```python
from build123d import *

# Parameters (mm, degrees)
BOSS_EXTRUDE1_DEPTH = 200
SKETCH2_W           = 11
SKETCH2_H           = 5
CUT_EXTRUDE1_DEPTH  = 10
FILLET1_R           = 9
MIRROR1_START       = 184
MIRROR1_DEPTH       = 11


with BuildPart() as part:
    # Sketch1 → Boss-Extrude1 (new body)
    with BuildSketch(Plane(origin=(0, 0, 0), x_dir=(0, 0, -1), z_dir=(1, 0, 0))):
        with BuildLine():
            Line((-9.5, 0), (-9.5, -9.5))
            ThreePointArc((-9.5, -9.5), (0, -19), (9.5, -9.5))
            Line((9.5, -9.5), (9.5, 0))
            ThreePointArc((9.5, 0), (0, 9.5), (-9.5, 0))
        make_face()
    extrude(amount=BOSS_EXTRUDE1_DEPTH)

    # Sketch2 → Cut-Extrude1 (cut, symmetric)
    with BuildSketch(Plane.XY):
        with Locations((10.5, -16.5)):
            Rectangle(SKETCH2_W, SKETCH2_H)
    extrude(amount=CUT_EXTRUDE1_DEPTH, both=True, mode=Mode.SUBTRACT)

    # Fillet1
    # the kernel refuses this fillet: 9 mm, written as the material it takes off along each edge
    with BuildSketch(Plane(origin=(16, -14, -8.366600265), x_dir=(0, 0.9921634898396948, -0.12494642623587741), z_dir=(-1, 0, 0))) as fillet1_piece_1:
        with BuildLine():
            CenterArc((7.946567819, -8.929471409), FILLET1_R, 82.822338024, 90)
            Line((-0.98290359, -7.804953572), (-1.875850731, -7.692501789))
            Line((-1.875850731, -7.692501789), (-0.892947141, 0.112451784))
            Line((-0.892947141, 0.112451784), (-0.323939264, 0.839680507))
            ThreePointArc((-0.323939264, 0.839680507), (4.718801734, 1.455206059), (9.183537439, 0.892947141))
            Line((9.183537439, 0.892947141), (9.071085655, 0))
        make_face()
    extrude(amount=11, mode=Mode.SUBTRACT)
    with BuildSketch(Plane(origin=(16, -14, 8.366600265), x_dir=(0, 0.9921634898396948, 0.1249464262358778), z_dir=(-1, 0, 0))) as fillet1_piece_2:
        with BuildLine():
            CenterArc((7.946567819, 8.929471409), FILLET1_R, 187.177661976, 90)
            Line((-0.98290359, 7.804953572), (-1.875850731, 7.692501789))
            Line((-1.875850731, 7.692501789), (-0.892947141, -0.112451784))
            Line((-0.892947141, -0.112451784), (-0.323939264, -0.839680507))
            ThreePointArc((-0.323939264, -0.839680507), (4.718801734, -1.455206059), (9.183537439, -0.892947141))
            Line((9.183537439, -0.892947141), (9.071085655, 0))
        make_face()
    extrude(amount=11, mode=Mode.SUBTRACT)

    # Mirror1: read off the stored shape, not the designer's step
    # Mirror1 outline → Mirror1 (cut)
    with BuildSketch(Plane.YZ.offset(MIRROR1_START)):
        with BuildLine():
            ThreePointArc((-5, -9.5), (-11.363961031, -6.863961031), (-14, -0.5))
            Line((-14, -0.5), (-14, 0.5))
            ThreePointArc((-14, 0.5), (-11.363961031, 6.863961031), (-5, 9.5))
            Line((-5, 9.5), (-9.5, 9.5))
            ThreePointArc((-9.5, 9.5), (-19, 0), (-9.5, -9.5))
            Line((-9.5, -9.5), (-5, -9.5))
        make_face()
    extrude(amount=MIRROR1_DEPTH, mode=Mode.SUBTRACT)


solid = part.part
```
Verification items for the finished model (mm, model axes). A direction names the side the tool comes from. Coordinates: 2 decimals unless noted, no trailing zeros. Loops run counter-clockwise (first coordinate to the right, second up) from the corner with the lowest first, then second, coordinate; pieces in that order, holes last. Notation, with made-up numbers: (58.25, -31.5) - (111.25, -31.5) arc R32 cw to (111.25, -5.5) - close; hole circle Ø2 at (16, 14). An arc over 180 degrees is marked (long way). Put each result on its own line as item: value.
Item 1: Section check B-B (z = 5.25). Enter the section's corners in (x, y), then the cut area to 3 significant figures.
Conclusion:
outline: (0, -17.42) - (5, -17.42) - (5, -12.64) - (16, -12.64) - (16, -17.42) - (184, -17.42) - (184, -12.64) - (195, -12.64) - (195, -17.42) - (200, -17.42) - (200, 7.92) - (0, 7.92) - close
area: 4,960 mm2
Item 2: Section check C-C (x = 62). Enter the section's corners in (y, z), then the cut area to 3 significant figures.
Conclusion:
outline: (-9.5, -9.5) - (0, -9.5) arc R9.5 ccw to (0, 9.5) - (-9.5, 9.5) arc R9.5 ccw to start
area: 464 mm2
Item 3: Set-up check for faces 4 (the face through (10.577, -11.294, -6.934)), 5 (the face through (16, -15, 0)), 6 (the face through (99, -5, 9.5)), 7 (the face through (189.423, -11.434, 6.794)): record each of +Z, -Z, +X, -X, +Y, -Y from which the full face is reachable in a straight line by a thin tool's end or side.
Conclusion:
face 4: -Z, -Y
face 5: -Y
face 6: +Z, +X, -X, +Y, -Y
face 7: +Z, -Y
Item 4: Gauge pin test, flat ends, axial feed: pin 1 Ø1.5 at (x, y) = (59.5, 3) entering from -Z; pin 2 Ø0.5 at (x, z) = (191.5, 0) entering from -Y; pin 3 Ø10 at (x, z) = (167, -5.5) entering from -Y. Record the tip position at first contact, or that the pin passes through.
Conclusion:
pin 1: stops at z = -9.23
pin 2: stops at y = -14
pin 3: stops at y = -18.99
Item 5: Draft check along X on faces 1 (the face through (99, -19, 0)), 2 (the face through (195, -15, 0)), 3 (the face through (200, -5, 0)). Enter one of: pulls with the +X half, pulls with the -X half, needs draft (parallel to the pull), parting line crosses it, or undercut.
Conclusion:
face 1: needs draft
face 2: undercut
face 3: pulls with the +X half
Item 6: Section check D-D (y = 6.5). Enter the section's corners in (x, z).
Conclusion:
outline: (0, -6.93) - (200, -6.93) - (200, 6.93) - (0, 6.93) - close
Item 7: Section check A-A (y = -16.5). Enter the section's corners in (x, z), then the cut area to 3 significant figures.
Conclusion:
outline: (0, -6.42) - (5, -6.42) - (5, 6.42) - (0, 6.42) - close; (16, -6.42) - (184, -6.42) - (184, 6.42) - (16, 6.42) - close; (195, -6.42) - (200, -6.42) - (200, 6.42) - (195, 6.42) - close
area: 2,290 mm2
Item 8: Scan lines: line 1 along X through (y, z) = (-12.25, 7); line 2 along Y through (x, z) = (61.5, 0.25); line 3 along Z through (x, y) = (171, 3.75). Record each from-to range of solid material in increasing order.
Conclusion:
line 1: x = 0 to 5, 16 to 184, 195 to 200
line 2: y = -19 to 9.5
line 3: z = -8.73 to 8.73
